from build123d import *

# Parameters (mm, degrees)
SKETCH1_W           = 51.260430681
SKETCH1_H           = 152.4
SKETCH1_R           = 6.35
BOSS_EXTRUDE1_DEPTH = 25.4
SKETCH6_R           = 2.0193
CUT_EXTRUDE4_DEPTH  = 25.4


with BuildPart() as part:
    # Sketch1 → Boss-Extrude1 (new body)
    with BuildSketch(Plane(origin=(0, 0, 0), x_dir=(0, 0, -1), z_dir=(1, 0, 0))):
        with Locations((-75.96978466, 76.2)):
            Rectangle(SKETCH1_W, SKETCH1_H)
        with Locations((-76.2, 50.8)):
            Circle(SKETCH1_R, mode=Mode.SUBTRACT)
        with Locations((-76.2, 69.85)):
            Circle(SKETCH1_R, mode=Mode.SUBTRACT)
        with Locations((-76.2, 88.9)):
            Circle(SKETCH1_R, mode=Mode.SUBTRACT)
        with Locations((-76.2, 107.95)):
            Circle(SKETCH1_R, mode=Mode.SUBTRACT)
        with Locations((-76.2, 127)):
            Circle(SKETCH1_R, mode=Mode.SUBTRACT)
    extrude(amount=BOSS_EXTRUDE1_DEPTH)

    # Sketch6 → Cut-Extrude4 (cut)
    with BuildSketch(Plane.XZ):
        with Locations(Location((12.7, 75.739569319, 0), (0, 0, 270))):
            Circle(SKETCH6_R)
    extrude(amount=-CUT_EXTRUDE4_DEPTH, mode=Mode.SUBTRACT)


solid = part.part
For this review, take the finished solid that the model builds, in its own axes (mm). A direction names the side the tool comes from. Give positions to 0.01 mm unless a question says otherwise; leave off trailing zeros. Order: outer loops, then holes, each group sorted by start corner. A loop starts at its lowest first (then second) coordinate and runs counter-clockwise, first axis right, second up. Notation, with made-up numbers: (27.25, 80.5) - (71.25, 80.5) arc R19 ccw to (71.25, 114.5) - close; hole circle Ø4 at (50.25, 52). An arc over 180 degrees is marked (long way). Answer as a JSON object with one key per item and string values. Group by question number.
Item 1: Take a section at B-B on y = 127. Give the boundary of the cut face in (x, z), and give its area (3 significant figures).
Item 2: Wall thickness on line 1 along Y through (x, z) = (8, 76.2); line 2 along Y through (x, z) = (7.25, 79.5); line 3 along Z through (x, y) = (14.75, 113.5): over which ranges is each line inside the solid? List them lowest first.
Item 3: Take a section at D-D on y = 105. Give the boundary of the cut face in (x, z), and give its area (3 significant figures).
Item 4: Draft analysis for pull direction Z (two halves, no side actions). For faces 3 (the flat face through (13, 75, 101.6)), 4 (the cylindrical face through (12.52, 55.09, 80.88)), 5 (the flat face through (13, 25.4, 76)), 6 (the flat face through (0, 77, 76)), state which applies: pulls with the +Z half, pulls with the -Z half, needs draft (parallel to the pull), parting line crosses it, or undercut.
Item 5: Machinability: for faces 1 (the cylindrical face through (11.927, 12.522, 73.874)), 2 (the flat face through (15, 0, 76)), which of the approach directions +Z, -Z, +X, -X, +Y, -Y give a long, thin tool a straight path to every point of the face, cutting with its end or side? Answer none if there is none.
Item 6: Take a section at A-A on x = 16.25. Give the boundary of the cut face in (y, z), and give its area (3 significant figures).
Item 7: Clearance check with flat-ended pins moving along their axes: pin 1 Ø16.5 at (y, z) = (107.95, 76.2) entering from -X; pin 2 Ø3.5 at (x, z) = (12.7, 75.74) entering from -Y; pin 3 Ø7.5 at (y, z) = (50.8, 76.2) entering from +X. State where each tip first meets the part, or that it passes through.
Item 8: Take a section at C-C on z = 76.2. Give the boundary of the cut face in (x, y).
Reported:
{
 "1": {"outline": "(0, 50.34) - (25.4, 50.34) - (25.4, 69.85) - (0, 69.85) - close; (0, 82.55) - (25.4, 82.55) - (25.4, 101.6) - (0, 101.6) - close", "area": "979 mm^2"},
 "2": {"line 1": "0 to 44.45, 57.15 to 63.5, 76.2 to 82.55, 95.25 to 101.6, 114.3 to 120.65, 133.35 to 152.4", "line 2": "0 to 45.37, 56.23 to 64.42, 75.28 to 83.47, 94.33 to 102.52, 113.38 to 121.57, 132.43 to 152.4", "line 3": "50.34 to 73.11, 79.29 to 101.6"},
 "3": {"outline": "(0, 50.34) - (25.4, 50.34) - (25.4, 70.58) - (0, 70.58) - close; (0, 81.82) - (25.4, 81.82) - (25.4, 101.6) - (0, 101.6) - close", "area": "1,020 mm^2"},
 "4": {"face 3": "pulls with the +Z half", "face 4": "undercut", "face 5": "undercut", "face 6": "needs draft"},
 "5": {"face 1": "-Y", "face 2": "+Z, -Z, +X, -X, -Y"},
 "6": {"outline": "(0, 50.34) - (152.4, 50.34) - (152.4, 101.6) - (0, 101.6) - close; hole circle Ø12.7 at (50.8, 76.2); hole circle Ø12.7 at (69.85, 76.2); hole circle Ø12.7 at (88.9, 76.2); hole circle Ø12.7 at (107.95, 76.2); hole circle Ø12.7 at (127, 76.2)", "area": "7,180 mm^2"},
 "7": {"pin 1": "x = 0", "pin 2": "y = 25.4", "pin 3": "through"},
 "8": {"outline": "(0, 0) - (10.73, 0) - (10.73, 25.4) - (14.67, 25.4) - (14.67, 0) - (25.4, 0) - (25.4, 44.45) - (0, 44.45) - close; (0, 57.15) - (25.4, 57.15) - (25.4, 63.5) - (0, 63.5) - close; (0, 76.2) - (25.4, 76.2) - (25.4, 82.55) - (0, 82.55) - close; (0, 95.25) - (25.4, 95.25) - (25.4, 101.6) - (0, 101.6) - close; (0, 114.3) - (25.4, 114.3) - (25.4, 120.65) - (0, 120.65) - close; (0, 133.35) - (25.4, 133.35) - (25.4, 152.4) - (0, 152.4) - close"}
}
